Build history of the part. All positions in model axes, mm. Coordinates: 2 decimals unless noted, no trailing zeros. Loops run counter-clockwise (first coordinate to the right, second up) from the corner with the lowest first, then second, coordinate; pieces in that order, holes last. Notation, with made-up numbers: (0, 42.25) - (4, 42.25) arc R18 ccw to (4, 47.25) - close; hole circle Ø10 at (9.5, 44.25). An arc over 180 degrees is marked (long way). One line per item, written item: value.
```python
from build123d import *

# Parameters (mm, degrees)
IZIM1_W                     = 25
IZIM1_H                     = 24.09
Y_KSEKLIK_EKSTR_ZYON1_DEPTH = 1.6
IZIM2_W                     = 17
IZIM2_H                     = 3.5
Y_KSEKLIK_EKSTR_ZYON2_DEPTH = 2
RADYUS1_R                   = 1
IZIM5_R                     = 1
KES_EKSTR_ZYON1_DEPTH       = 10


with BuildPart() as part:
    # Çizim1 → Yükseklik-Ekstrüzyon1 (new body)
    with BuildSketch(Plane(origin=(1.6, 0, 0), x_dir=(0, 0, -1), z_dir=(1, 0, 0))):
        with Locations((0, -5.455)):
            Rectangle(IZIM1_W, IZIM1_H)
    extrude(amount=-Y_KSEKLIK_EKSTR_ZYON1_DEPTH)

    # Çizim2 → Yükseklik-Ekstrüzyon2 (add)
    with BuildSketch(Plane(origin=(1.6, 0, 0), x_dir=(0, 0, -1), z_dir=(1, 0, 0))):
        with Locations((0, -15.25)):
            Rectangle(IZIM2_W, IZIM2_H)
    extrude(amount=Y_KSEKLIK_EKSTR_ZYON2_DEPTH)

    # Radyus1
    radyus1_edges = [part.edges().sort_by_distance(p)[0] for p in [
        (0.8, 6.59, -12.5),
        (0.8, -17.5, -12.5),
        (0.8, -17.5, 12.5),
        (0.8, 6.59, 12.5),
    ]]
    fillet(radyus1_edges, radius=RADYUS1_R)

    # Çizim5 → Kes-Ekstrüzyon1 (cut)
    with BuildSketch(Plane(origin=(1.6, 0, 0), x_dir=(0, 0, -1), z_dir=(1, 0, 0))):
        with Locations((10.5, 4.59)):
            Circle(IZIM5_R)
        with Locations((-10.5, 4.59)):
            Circle(IZIM5_R)
        with Locations((-10.5, -8)):
            Circle(IZIM5_R)
        with Locations((10.5, -8)):
            Circle(IZIM5_R)
    extrude(amount=-KES_EKSTR_ZYON1_DEPTH, mode=Mode.SUBTRACT)


solid = part.part
```
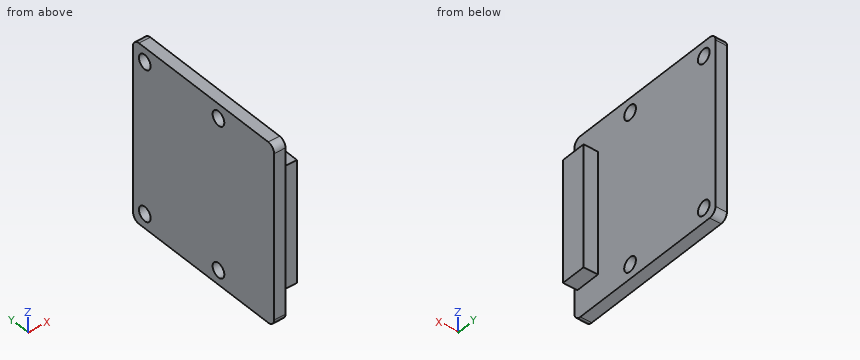
Item 1: Probe probe 1 along X at (y, z) = (-15.75, 9.75); probe 2 along Y at (x, z) = (2.5, -4.25). List the from-to ranges inside material, lowest first. Write a range as from..to.
Check result:
probe 1: x = 0..1.6
probe 2: y = -17..-13.5
Item 2: Cut at B-B, the plane x = 1.15. Write the cut outline in (y, z), then the cut area to 3 significant figures.
Check result:
outline: (-17.5, -11.5) arc R1 ccw to (-16.5, -12.5) - (5.59, -12.5) arc R1 ccw to (6.59, -11.5) - (6.59, 11.5) arc R1 ccw to (5.59, 12.5) - (-16.5, 12.5) arc R1 ccw to (-17.5, 11.5) - close; hole circle Ø2 at (-8, -10.5); hole circle Ø2 at (-8, 10.5); hole circle Ø2 at (4.59, -10.5); hole circle Ø2 at (4.59, 10.5)
area: 589 mm^2
Item 3: Cut at C-C, the plane y = -8. Write the cut outline in (x, z), then the cut area to 3 significant figures.
Check result:
outline: (0, -12.5) - (1.6, -12.5) - (1.6, -11.5) - (0, -11.5) - close; (0, -9.5) - (1.6, -9.5) - (1.6, 9.5) - (0, 9.5) - close; (0, 11.5) - (1.6, 11.5) - (1.6, 12.5) - (0, 12.5) - close
area: 33.6 mm^2
Item 4: Drop flat-ended pins along their axis: P1, Ø8, axis at y = -14.5, z = -4, coming from the -X side; P2, Ø3, axis at y = -3.5, z = 5, coming from the +X side; P3, Ø1, axis at x = 3, y = -16, coming from the -Z side. Give the stop position or say it passes through.
Check result:
P1: stops at x = 0
P2: stops at x = 1.6
P3: stops at z = -8.5
Item 5: Cut at A-A, the plane z = -10.5. Write the cut outline in (x, y).
Check result:
outline: (0, -17.5) - (1.6, -17.5) - (1.6, -9) - (0, -9) - close; (0, -7) - (1.6, -7) - (1.6, 3.59) - (0, 3.59) - close; (0, 5.59) - (1.6, 5.59) - (1.6, 6.59) - (0, 6.59) - close
Item 6: Cut at D-D, the plane z = -6.5. Write the cut outline in (x, y), then the cut area to 3 significant figures.
Check result:
outline: (0, -17.5) - (1.6, -17.5) - (1.6, -17) - (3.6, -17) - (3.6, -13.5) - (1.6, -13.5) - (1.6, 6.59) - (0, 6.59) - close
area: 45.5 mm^2
